from build123d import *

# Parameters (mm, degrees)
SKETCH_1_R      = 5
SKETCH_1_W      = 4.5
SKETCH_1_H      = 47
SKETCH_1_R_2    = 1.15
EXTRUDE_1_DEPTH = 10
FILLET_1_R      = 1.5


with BuildPart() as part:
    # 草图1 → 凸台-拉伸1 (new, symmetric)
    # profile 1 of 2: a face of its own
    with BuildSketch(Plane.XY):
        with Locations((0, -23.5)):
            Circle(SKETCH_1_R)
    # profile 2 of 2: a face of its own
    with BuildSketch(Plane.XY):
        Rectangle(SKETCH_1_W, SKETCH_1_H)
        with Locations((0, -0.5)):
            Circle(SKETCH_1_R_2, mode=Mode.SUBTRACT)
        with Locations((0, 14.5)):
            Circle(SKETCH_1_R_2, mode=Mode.SUBTRACT)
        with Locations((0, 21.5)):
            Circle(SKETCH_1_R_2, mode=Mode.SUBTRACT)
    extrude(amount=EXTRUDE_1_DEPTH, both=True)

    # 圆角1
    fillet_1_edges = [part.edges().sort_by_distance(p)[0] for p in [
        (-2.25, 23.5, 0),
        (2.25, 23.5, 0),
    ]]
    fillet(fillet_1_edges, radius=FILLET_1_R)


solid = part.part
CAD build for the part. Positions are in the model's coordinates, mm. A direction names the side the tool comes from. Round coordinates to 2 decimals unless told otherwise and drop trailing zeros. Loops run counter-clockwise (first coordinate to the right, second up) from the corner with the lowest first, then second, coordinate; pieces in that order, holes last. Notation, with made-up numbers: (-37.5, -26.75) - (-23.5, -26.75) arc R27 cw to (-23.5, 2.25) - close; hole circle Ø3 at (-1, 56). An arc over 180 degrees is marked (long way). Put each result on its own line as item: value.
1. Pin check, flat tips, straight feed: P1, Ø1.4, axis at x = 0, y = -0.5, coming from the -Z side; P2, Ø6, axis at y = 8, z = 7, coming from the -X side; P3, Ø6, axis at x = -3.5, y = -11.5, coming from the -Z side; P4, Ø1, axis at x = -2.5, z = -3, coming from the +Y side. Stop position of each tip, or through.
Geometry check:
P1: through
P2: x = -2.25
P3: z = -10
P4: y = 22.83
2. Slice it at B-B on y = 21.5. List the corners of the cut face in (x, z), and give its area (3 significant figures).
Geometry check:
outline: (-2.25, -10) - (-1.15, -10) - (-1.15, 10) - (-2.25, 10) - close; (1.15, -10) - (2.25, -10) - (2.25, 10) - (1.15, 10) - close
area: 44.0 mm²
3. Wall check: line 1 (Y direction, x = 0, z = 7); line 2 (X direction, y = 6.5, z = -7.25); line 3 (Y direction, x = 3.75, z = -0.75). Give the ranges that are in metal, low to high.
Geometry check:
line 1: -28.5 to -1.65, 0.65 to 13.35, 15.65 to 20.35, 22.65 to 23.5
line 2: -2.25 to 2.25
line 3: -26.81 to -20.19
4. Slice it at C-C on z = -1.5. List the corners of the cut face in (x, y), and give its area (3 significant figures).
Geometry check:
outline: (-2.25, -19.03) arc R5 ccw (long way) to (2.25, -19.03) - (2.25, 22) arc R1.5 ccw to (0.75, 23.5) - (-0.75, 23.5) arc R1.5 ccw to (-2.25, 22) - close; hole circle Ø2.3 at (0, -0.5); hole circle Ø2.3 at (0, 14.5); hole circle Ø2.3 at (0, 21.5)
area: 255 mm²
5. Slice it at D-D on y = -11. List the corners of the cut face in (x, z), and give its area (3 significant figures).
Geometry check:
outline: (-2.25, -10) - (2.25, -10) - (2.25, 10) - (-2.25, 10) - close
area: 90.0 mm²
6. 3-axis set-ups, long thin cutter, end or side, ignore diameter. For faces 1 (the flat face through (-2.25, 1, 0)), 2 (the flat face through (0, -8, -10)), 3 (the flat face through (2.25, 1, 0)): which of +Z, -Z, +X, -X, +Y, -Y reach the whole face in a straight line?
Geometry check:
face 1: +Z, -Z, -X, +Y
face 2: -Z, +X, -X, +Y, -Y
face 3: +Z, -Z, +X, +Y
7. Slice it at A-A on x = 0. List the corners of the cut face in (y, z), and give its area (3 significant figures).
Geometry check:
outline: (-28.5, -10) - (-1.65, -10) - (-1.65, 10) - (-28.5, 10) - close; (0.65, -10) - (13.35, -10) - (13.35, 10) - (0.65, 10) - close; (15.65, -10) - (20.35, -10) - (20.35, 10) - (15.65, 10) - close; (22.65, -10) - (23.5, -10) - (23.5, 10) - (22.65, 10) - close
area: 902 mm²
